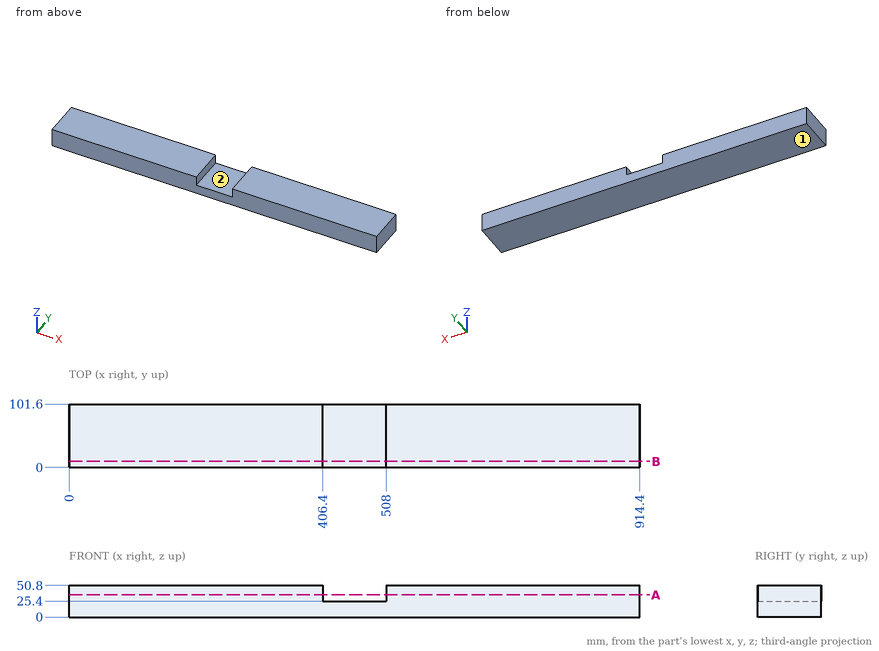
Design review of the part shown in the three views and the two pictorial views. Dimensions are in mm from the part's minimum x, y and z. Give positions to 0.01 mm unless a question says otherwise; leave off trailing zeros. Write each loop counter-clockwise with the first axis right and the second up, starting at its lowest first coordinate (ties: lowest second). Pieces come first, ordered by that corner, then holes.
(1) Mouldability with a two-part tool opening along X and no side actions: class the marked faces 1 and 2 as +X half, -X half, draft (parallel to the pull), parting line (faces both ways), or undercut.
Checked values:
face 1: draft
face 2: undercut
(2) Add section B-B (y = 9.5). Give the boundary of the cut face in (x, z), and give its area (3 significant figures).
Checked values:
outline: (0, 0) - (914.4, 0) - (914.4, 50.8) - (508, 50.8) - (508, 25.4) - (406.4, 25.4) - (406.4, 50.8) - (0, 50.8) - close
area: 43,900 mm2
(3) Add section A-A (z = 35.5). Give the boundary of the cut face in (x, y), and give its area (3 significant figures).
Checked values:
outline: (0, 0) - (406.4, 0) - (406.4, 101.6) - (0, 101.6) - close; (508, 0) - (914.4, 0) - (914.4, 101.6) - (508, 101.6) - close
area: 82,600 mm2
(4) Clearance check with a flat-ended pin moving along its axis: pin 1 Ø1.5 at (y, z) = (89.5, 28.5) entering from -X. State where the tip first meets the part, or that it passes through.
Checked values:
pin 1: stops at x = 0
(5) Wall thickness on line 1 along X through (y, z) = (86, 36.5); line 2 along Z through (x, y) = (464, 54.5): over which ranges is each line inside the solid? List them lowest first.
Checked values:
line 1: x = 0 to 406.4, 508 to 914.4
line 2: z = 0 to 25.4
